The figure shows three views and two pictorial views of one solid part (mm, origin at its lowest corner). Answer the questions. A direction names the side the tool comes from. Give positions to 0.01 mm unless a question says otherwise; leave off trailing zeros. Write each loop counter-clockwise with the first axis right and the second up, starting at its lowest first coordinate (ties: lowest second). Pieces come first, ordered by that corner, then holes. Notation, with made-up numbers: (45.5, 51.5) -> (88.5, 51.5) arc R21 cw to (88.5, 63.5) -> close; hole circle Ø3 at (0.25, -16.5). An arc over 180 degrees is marked (long way). Answer as CSV lines item,"result". Start each with the question number.
1. A tool of negligible diameter and unlimited length cuts with its end or side. For the marked faces 1, 2 and 3, from which of +Z, -Z, +X, -X, +Y, -Y can it reach the whole face along a straight path? Write none if from no direction.
2. Given pin 1 (2.5 mm diameter, centred on x = 111, y = 105, fed in from +Z); pin 2 (14.5 mm diameter, centred on x = 59.5, y = 9.5, fed in from -Z); pin 3 (10 mm diameter, centred on x = 89.5, z = 6.5, fed in from +Y), each flat-ended and moving along its own axis, determine where each tip first touches the part or whether it passes through.
3. The part is cut by section C-C, the plane y = 105. Determine the outline of the cut face in (x, z), and give its area (3 significant figures).
4. The part is cut by section D-D, the plane y = 13.5. Determine the outline of the cut face in (x, z).
5. The part is cut by section B-B, the plane x = 81.5. Determine the outline of the cut face in (y, z).
6. Find the intervals of material crossed by line 1 (Y direction, x = 13, z = 8); line 2 (Y direction, x = 80.5, z = 32.5); line 3 (X direction, y = 52.5, z = 19), in increasing order.
7. The part is cut by section A-A, the plane z = 10. Determine the outline of the cut face in (x, y).
8. For a pull along Y with two mould halves and no side action, classify the marked faces 4, 5, 6 and 7 as pulls with the +Y half, pulls with the -Y half, needs draft (parallel to the pull), parting line crosses it, or undercut.
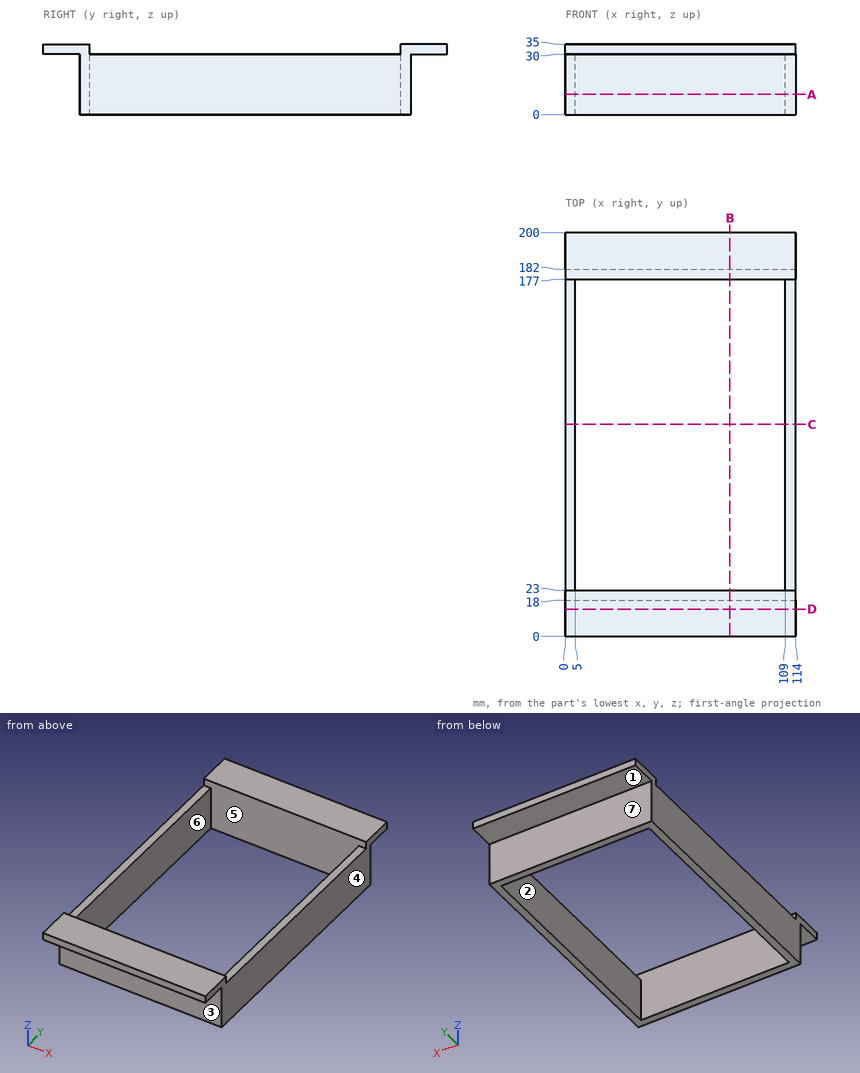
Results found:
1,face 1,"-Z, +X, -X, +Y"
1,face 2,"+Z, -Z"
1,face 3,"-Z, +X, -X, -Y"
2,pin 1,"stops at z = 30"
2,pin 2,"stops at z = 30"
2,pin 3,"stops at y = 182"
3,outline,"(0, 0) -> (5, 0) -> (5, 30) -> (0, 30) -> close; (109, 0) -> (114, 0) -> (114, 30) -> (109, 30) -> close"
3,area,"300 mm²"
4,outline,"(0, 30) -> (114, 30) -> (114, 35) -> (0, 35) -> close"
5,outline,"(0, 30) -> (18, 30) -> (18, 0) -> (23, 0) -> (23, 35) -> (0, 35) -> close; (177, 0) -> (182, 0) -> (182, 30) -> (200, 30) -> (200, 35) -> (177, 35) -> close"
6,line 1,"y = 18 to 23, 177 to 182"
6,line 2,"y = 0 to 23, 177 to 200"
6,line 3,"x = 0 to 5, 109 to 114"
7,outline,"(0, 18) -> (114, 18) -> (114, 182) -> (0, 182) -> close; hole (5, 23) -> (109, 23) -> (109, 177) -> (5, 177) -> close"
8,face 4,"needs draft"
8,face 5,"undercut"
8,face 6,"undercut"
8,face 7,"pulls with the +Y half"
